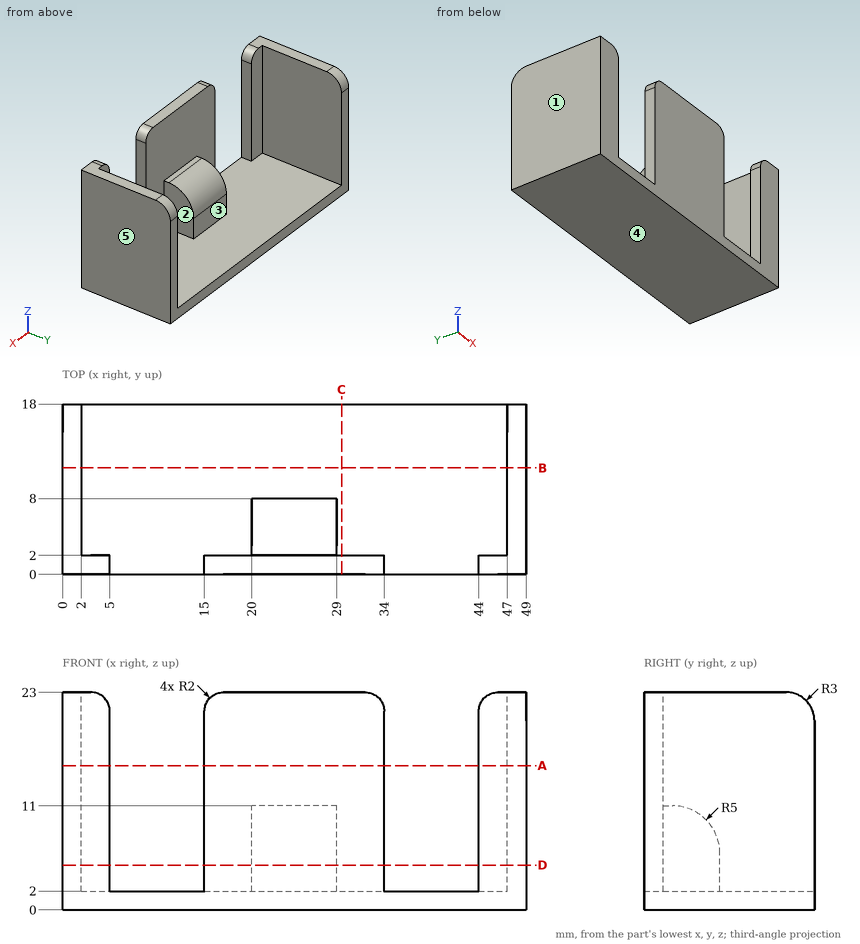
Check sheet for the drawn part. Datum: minimum x, y, z corner. Units: mm. A direction names the side the tool comes from. Coordinates: 2 decimals unless noted, no trailing zeros. Loops run counter-clockwise (first coordinate to the right, second up) from the corner with the lowest first, then second, coordinate; pieces in that order, holes last. Notation, with made-up numbers: (29.25, 38.5) -> (86.25, 38.5) arc R18 cw to (86.25, 53.5) -> close; hole circle Ø7 at (50.5, 29). An arc over 180 degrees is marked (long way). Answer in a Markdown table with one row per item.
1. Sectioned sample at B-B, the plane y = 11.25. Record the boundary of the cut face in (x, z), then the cut area to 3 significant figures.
Check values:
| item | result |
|---|---|
| outline | (0, 0) -> (49, 0) -> (49, 23) -> (47, 23) -> (47, 2) -> (2, 2) -> (2, 23) -> (0, 23) -> close |
| area | 182 mm2 |
2. Access from +Z, -Z, +X, -X, +Y, -Y to the whole of each face (thin tool, end or side, straight path). Record for the marked faces 1 and 2.
Check values:
| item | result |
|---|---|
| face 1 | +Z, -Z, -X, +Y, -Y |
| face 2 | +Z, +Y |
3. Sectioned sample at D-D, the plane z = 4.75. Record the boundary of the cut face in (x, y).
Check values:
| item | result |
|---|---|
| outline | (0, 0) -> (5, 0) -> (5, 2) -> (2, 2) -> (2, 18) -> (0, 18) -> close; (15, 0) -> (34, 0) -> (34, 2) -> (29, 2) -> (29, 8) -> (20, 8) -> (20, 2) -> (15, 2) -> close; (44, 0) -> (49, 0) -> (49, 18) -> (47, 18) -> (47, 2) -> (44, 2) -> close |
4. Release check for a two-part mould opening along X. For the marked faces 3, 4 and 5 record: released by +X, released by -X, zero draft, split by the parting line, or undercut.
Check values:
| item | result |
|---|---|
| face 3 | undercut |
| face 4 | zero draft |
| face 5 | released by +X |
5. Material ranges on line 1 along X through (y, z) = (11.75, 10); line 2 along Z through (x, y) = (32.5, 9.5), recorded low to high. Write a range as [from, to].
Check values:
| item | result |
|---|---|
| line 1 | x = [0, 2], [47, 49] |
| line 2 | z = [0, 2] |
6. Sectioned sample at A-A, the plane z = 15.25. Record the boundary of the cut face in (x, y), then the cut area to 3 significant figures.
Check values:
| item | result |
|---|---|
| outline | (0, 0) -> (5, 0) -> (5, 2) -> (2, 2) -> (2, 18) -> (0, 18) -> close; (15, 0) -> (34, 0) -> (34, 2) -> (15, 2) -> close; (44, 0) -> (49, 0) -> (49, 18) -> (47, 18) -> (47, 2) -> (44, 2) -> close |
| area | 122 mm2 |
7. Go/stop test with flat-tipped pins: pin 1 (5.5 mm diameter, centred on x = 28.5, z = 9.5, fed in from +Y); pin 2 (0.5 mm diameter, centred on x = 24.5, y = 2.5, fed in from +Z); pin 3 (4.5 mm diameter, centred on x = 26, z = 4.5, fed in from +Y). Record where each tip stops, or that it passes through.
Check values:
| item | result |
|---|---|
| pin 1 | stops at y = 7.94 |
| pin 2 | stops at z = 11 |
| pin 3 | stops at y = 8 |
8. Sectioned sample at C-C, the plane x = 29.5. Record the boundary of the cut face in (y, z), then the cut area to 3 significant figures.
Check values:
| item | result |
|---|---|
| outline | (0, 0) -> (18, 0) -> (18, 2) -> (2, 2) -> (2, 23) -> (0, 23) -> close |
| area | 78.0 mm2 |
